from build123d import *

# Parameters (mm, degrees)
BASE_EXTRUDE_DEPTH  = 0.9906
SKETCH8_R           = 1.524
CUT_EXTRUDE4_DEPTH  = 27.808529889
BOSS_EXTRUDE5_DEPTH = 16.8148
FILLET3_R           = 0.508
CUT_EXTRUDE5_DEPTH  = 15.8054
LPATTERN1_COUNT     = 2
LPATTERN1_PITCH     = 16


with BuildPart() as part:
    # Sketch1 → Base-Extrude (new body)
    with BuildSketch(Plane.XY):
        with BuildLine():
            Line((-13.6498, 6.2738), (13.6498, 6.2738))
            ThreePointArc((13.6498, 6.2738), (14.781312271, 5.805112271), (15.25, 4.6736))
            Line((15.25, 4.6736), (15.25, -20.426))
            ThreePointArc((15.25, -20.426), (14.781312271, -21.557512271), (13.6498, -22.0262))
            Line((13.6498, -22.0262), (-13.6498, -22.0262))
            ThreePointArc((-13.6498, -22.0262), (-14.781312271, -21.557512271), (-15.25, -20.426))
            Line((-15.25, -20.426), (-15.25, 4.6736))
            ThreePointArc((-15.25, 4.6736), (-14.781312271, 5.805112271), (-13.6498, 6.2738))
        make_face()
    extrude(amount=-BASE_EXTRUDE_DEPTH)

    # Sketch8 → Cut-Extrude4 (cut, through all)
    with BuildSketch(Plane.XY):
        with Locations((12.5, 0)):
            Circle(SKETCH8_R)
        with Locations(Location((-12.5, 0, 0), (0, 0, 180))):
            Circle(SKETCH8_R)
    cut_extrude4 = extrude(amount=-CUT_EXTRUDE4_DEPTH, mode=Mode.SUBTRACT)

    # Sketch14 → Boss-Extrude5 (add)
    with BuildSketch(Plane(origin=(0, 0, -0.9906), x_dir=(-1, 0, 0), z_dir=(0, 0, -1))):
        with BuildLine():
            Line((-10.5, 3.0738), (-10.5, -21.841863832))
            Line((-10.5, -21.841863832), (10.5, -21.841863832))
            Line((10.5, -21.841863832), (10.5, 3.0738))
            ThreePointArc((10.5, 3.0738), (9.621320344, 5.195120344), (7.5, 6.0738))
            Line((7.5, 6.0738), (-7.5, 6.0738))
            ThreePointArc((-7.5, 6.0738), (-9.621320344, 5.195120344), (-10.5, 3.0738))
        make_face()
    extrude(amount=BOSS_EXTRUDE5_DEPTH)

    # Fillet3
    fillet3_edges = [part.edges().sort_by_distance(p)[0] for p in [
        (-9.621320344, 5.195120344, -17.8054),
        (9.621320344, 5.195120344, -17.8054),
        (-10.5, -9.384031916, -17.8054),
        (0, 6.0738, -17.8054),
        (10.5, -9.384031916, -17.8054),
    ]]
    fillet(fillet3_edges, radius=FILLET3_R)

    # Sketch15 → Cut-Extrude5 (cut)
    with BuildSketch(Plane.XY):
        with BuildLine():
            Line((9.9, -21.0262), (-9.9, -21.0262))
            Line((-9.9, -21.0262), (-9.9, 3.0738))
            ThreePointArc((-9.9, 3.0738), (-9.197056275, 4.770856275), (-7.5, 5.4738))
            Line((-7.5, 5.4738), (7.5, 5.4738))
            ThreePointArc((7.5, 5.4738), (9.197056275, 4.770856275), (9.9, 3.0738))
            Line((9.9, 3.0738), (9.9, -21.0262))
        make_face()
    extrude(amount=-CUT_EXTRUDE5_DEPTH, mode=Mode.SUBTRACT)

    # LPattern1: Cut-Extrude4 ×2
    with Locations(*[(0, -i * LPATTERN1_PITCH, 0) for i in range(1, LPATTERN1_COUNT)]):
        add(cut_extrude4, mode=Mode.SUBTRACT)


solid = part.part
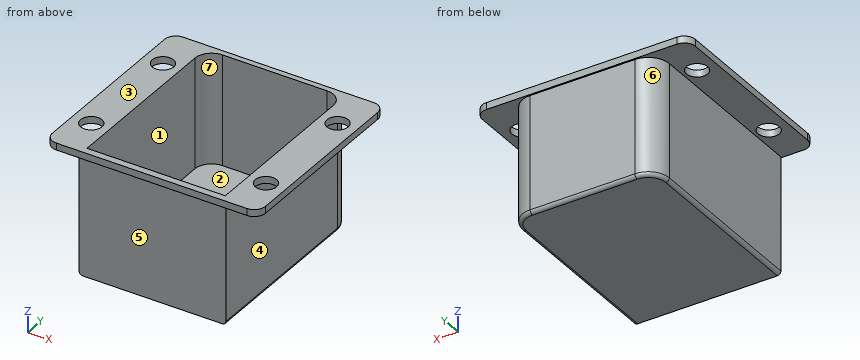
Geometry check sheet. Reference: the model listing, model coordinates, mm. Face numbers are marked on the shaded views. A direction names the side the tool comes from. Round coordinates to 2 decimals unless told otherwise and drop trailing zeros. Loops run counter-clockwise (first coordinate to the right, second up) from the corner with the lowest first, then second, coordinate; pieces in that order, holes last.
Item 1: Cross-section at B-B on y = 0. Record the boundary of the cut face in (x, z).
Item 2: Cross-section at A-A on x = 12.5. Record the boundary of the cut face in (y, z).
Item 3: Gauge pin test, flat ends, axial feed: pin 1 (1 mm diameter, centred on y = -7, z = -15, fed in from +X); pin 2 (3.5 mm diameter, centred on x = -12.5, y = 0, fed in from +Z); pin 3 (6 mm diameter, centred on x = 6.5, y = -16, fed in from +Z); pin 4 (1.5 mm diameter, centred on x = -7, z = -15, fed in from +Y). Record the tip position at first contact, or that the pin passes through.
Item 4: Thickness scan on line 1 (Y direction, x = 12.5, z = -0.2); line 2 (Y direction, x = 5, z = -15.75); line 3 (X direction, y = -14.5, z = -7.5). Record the ranges inside material, lowest first.
Item 5: Mould release check, pull along X, two halves, no side actions. Record for the marked faces 1, 2, 3 and 4: pulls with the +X half, pulls with the -X half, needs draft (parallel to the pull), parting line crosses it, or undercut.
Item 6: Cross-section at D-D on x = 0.5. Record the boundary of the cut face in (y, z).
Item 7: Access from +Z, -Z, +X, -X, +Y, -Y to the whole of each face (thin tool, end or side, straight path). Record for the marked faces 5, 6 and 7.
Item 8: Cross-section at C-C on z = -7.5. Record the boundary of the cut face in (x, y), then the cut area to 3 significant figures.
Answer sheet:
1. outline: (-15.25, -0.99) - (-14.02, -0.99) - (-14.02, 0) - (-15.25, 0) - close; (-10.98, -0.99) - (-10.5, -0.99) - (-10.5, -17.3) arc R0.51 ccw to (-9.99, -17.81) - (9.99, -17.81) arc R0.51 ccw to (10.5, -17.3) - (10.5, -0.99) - (10.98, -0.99) - (10.98, 0) - (9.9, 0) - (9.9, -15.81) - (-9.9, -15.81) - (-9.9, 0) - (-10.98, 0) - close; (14.02, -0.99) - (15.25, -0.99) - (15.25, 0) - (14.02, 0) - close
2. outline: (-22.03, -0.99) - (-17.52, -0.99) - (-17.52, 0) - (-22.03, 0) - close; (-14.48, -0.99) - (-1.52, -0.99) - (-1.52, 0) - (-14.48, 0) - close; (1.52, -0.99) - (6.27, -0.99) - (6.27, 0) - (1.52, 0) - close
3. pin 1: stops at x = 10.5
3. pin 2: stops at z = 0
3. pin 3: stops at z = -15.81
3. pin 4: stops at y = 6.07
4. line 1: y = -22.03 to -17.52, -14.48 to -1.52, 1.52 to 6.27
4. line 2: y = -21.84 to -21.03, 5.47 to 6.07
4. line 3: x = -10.5 to -9.9, 9.9 to 10.5
5. face 1: undercut
5. face 2: undercut
5. face 3: needs draft
5. face 4: pulls with the +X half
6. outline: (-22.03, -0.99) - (-21.84, -0.99) - (-21.84, -17.81) - (5.57, -17.81) arc R0.51 ccw to (6.07, -17.3) - (6.07, -0.99) - (6.27, -0.99) - (6.27, 0) - (5.47, 0) - (5.47, -15.81) - (-21.03, -15.81) - (-21.03, 0) - (-22.03, 0) - close
7. face 5: -Z, +X, -X, -Y
7. face 6: -Z, -X, +Y
7. face 7: +Z
8. outline: (-10.5, -21.84) - (10.5, -21.84) - (10.5, 3.07) arc R3 ccw to (7.5, 6.07) - (-7.5, 6.07) arc R3 ccw to (-10.5, 3.07) - close; hole (-9.9, -21.03) - (9.9, -21.03) - (9.9, 3.07) arc R2.4 ccw to (7.5, 5.47) - (-7.5, 5.47) arc R2.4 ccw to (-9.9, 3.07) - close
8. area: 60.1 mm2
